```python
from build123d import *

# Parameters (mm, degrees)
F0_W     = 40
F0_H     = 20
F0_R     = 2
F0_R_2   = 7
F0_R_3   = 5
F1_DEPTH = 3
F2_DEPTH = 15
F3_R     = 5


with BuildPart() as f1:
    # F0 (on Top) → F1 (new body)
    with BuildSketch(Plane.XY):
        Rectangle(F0_W, F0_H)
        with Locations((-15, 0)):
            Circle(F0_R, mode=Mode.SUBTRACT)
        Circle(F0_R_2, mode=Mode.SUBTRACT)
        with Locations((15, 0)):
            Circle(F0_R, mode=Mode.SUBTRACT)
        Circle(F0_R_2)
        Circle(F0_R_3, mode=Mode.SUBTRACT)
    extrude(amount=F1_DEPTH)

    # F0 (on Top) → F2 (join)
    with BuildSketch(Plane.XY):
        Circle(F0_R_2)
        Circle(F0_R_3, mode=Mode.SUBTRACT)
    extrude(amount=F2_DEPTH)

    # F3
    f3_edges = [f1.edges().sort_by_distance(p)[0] for p in [
        (-20, 10, 1.5),
        (-20, -10, 1.5),
        (20, -10, 1.5),
        (20, 10, 1.5),
    ]]
    fillet(f3_edges, radius=F3_R)


solid = f1.part
```
Input: part model. Units: mm. Frame: model coordinates. A direction names the side the tool comes from. Give positions to 0.01 mm unless a question says otherwise; leave off trailing zeros. Order: outer loops, then holes, each group sorted by start corner. A loop starts at its lowest first (then second) coordinate and runs counter-clockwise, first axis right, second up.
1. Line query: probe 1 along Y at (x, z) = (15, 2.35); probe 2 along Z at (x, y) = (18, -8.5); probe 3 along X at (y, z) = (2.5, 10.25). Output: solid intervals per line, ascending.
Computed:
probe 1: y = -10 to -2, 2 to 10
probe 2: z = 0 to 3
probe 3: x = -6.54 to -4.33, 4.33 to 6.54
2. Draft query along X for faces 3 (the face through (-18, -9, 2)), 4 (the face through (13.4, -1.2, 1.5)), 5 (the face through (0, -10, 1)). Return one class per face: released by +X, released by -X, zero draft, split by the parting line, or undercut.
Computed:
face 3: released by -X
face 4: undercut
face 5: zero draft
3. Cut plane A-A (x = 0). Return loops of the section in (y, z), and give its area (3 significant figures).
Computed:
outline: (-10, 0) - (-5, 0) - (-5, 15) - (-7, 15) - (-7, 3) - (-10, 3) - close; (5, 0) - (10, 0) - (10, 3) - (7, 3) - (7, 15) - (5, 15) - close
area: 78.0 mm2
4. Cut plane B-B (y = 0). Return loops of the section in (x, z), and give its area (3 significant figures).
Computed:
outline: (-20, 0) - (-17, 0) - (-17, 3) - (-20, 3) - close; (-13, 0) - (-5, 0) - (-5, 15) - (-7, 15) - (-7, 3) - (-13, 3) - close; (5, 0) - (13, 0) - (13, 3) - (7, 3) - (7, 15) - (5, 15) - close; (17, 0) - (20, 0) - (20, 3) - (17, 3) - close
area: 114 mm2
5. Set-up query: faces 1 (the face through (6.466, -2.681, 8.916)), 2 (the face through (-2, 5, 15)). Return all of +Z, -Z, +X, -X, +Y, -Y with unobstructed straight access to the full face (end or side cutting, diameter ignored); none if empty.
Computed:
face 1: +Z
face 2: +Z, +X, -X, +Y, -Y
6. Pin query (flat end, axial travel): pin 1 Ø5 at (x, y) = (15, 0) entering from +Z; pin 2 Ø3.5 at (x, y) = (-15, 0) entering from -Z; pin 3 Ø5 at (x, z) = (-1, 10.5) entering from -Y; pin 4 Ø4 at (x, y) = (8.5, 6) entering from -Z. Return the tip coordinate at first contact, or that it passes through.
Computed:
pin 1: stops at z = 3
pin 2: passes through
pin 3: stops at y = -7
pin 4: stops at z = 0
7. Cut plane D-D (y = 2.5). Return loops of the section in (x, z), and give its area (3 significant figures).
Computed:
outline: (-20, 0) - (-4.33, 0) - (-4.33, 15) - (-6.54, 15) - (-6.54, 3) - (-20, 3) - close; (4.33, 0) - (20, 0) - (20, 3) - (6.54, 3) - (6.54, 15) - (4.33, 15) - close
area: 147 mm2
8. Cut plane C-C (z = 1.5). Return loops of the section in (x, y), and give its area (3 significant figures).
Computed:
outline: (-20, -5) arc R5 ccw to (-15, -10) - (15, -10) arc R5 ccw to (20, -5) - (20, 5) arc R5 ccw to (15, 10) - (-15, 10) arc R5 ccw to (-20, 5) - close; hole circle Ø4 at (-15, 0); hole circle Ø10 at (0, 0); hole circle Ø4 at (15, 0)
area: 675 mm2
